```python
from build123d import *

# Parameters (mm, degrees)
F1_DEPTH = 20
F3_DEPTH = 20


with BuildPart() as f1:
    # F0 (on Top) → F1 (new body)
    with BuildSketch(Plane.XY):
        Polygon((0, 40), (0, 0), (20, 0), (20, 20), (40, 20), (40, 40), align=None)
    extrude(amount=F1_DEPTH)

    # F2 (on face) → F3 (join)
    with BuildSketch(Plane.XY.offset(20)):
        Polygon((0, 20), (20, 20), (40, 40), (0, 40), align=None)
    extrude(amount=F3_DEPTH)


solid = f1.part
```
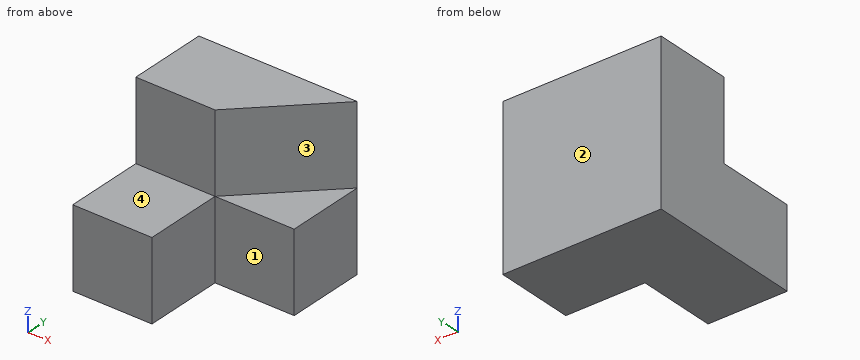
Could you check a few things on this model? Use its own coordinates, in mm. Face numbers are marked on the shaded views. A direction names the side the tool comes from. Give positions to 0.01 mm unless a question says otherwise; leave off trailing zeros. Write each loop counter-clockwise with the first axis right and the second up, starting at its lowest first coordinate (ties: lowest second). Pieces come first, ordered by that corner, then holes. Notation, with made-up numbers: (41, -7) - (67, -7) arc R25 ccw to (67, 21) - close; hole circle Ø8 at (50, 10.5). An arc over 180 degrees is marked (long way). One line per item, written item: value. Start each with the question number.
Item 1: Imagine slicing it at B-B, the plane x = 13. List the corners of the cut face in (y, z) for me, and give its area (3 significant figures).
Item 2: Imagine slicing it at D-D, the plane y = 12. List the corners of the cut face in (x, z) for me.
Item 3: Imagine slicing it at A-A, the plane y = 35. List the corners of the cut face in (x, z) for me.
Item 4: I'm going to push flat-ended pins straight in: pin 1 (6 mm diameter, centred on x = 7, z = 31, fed in from -Y); pin 2 (2 mm diameter, centred on y = 25, z = 25, fed in from +X); pin 3 (6 mm diameter, centred on y = 8, z = 12.5, fed in from +X). Where does each tip first touch, or does it pass through?
Item 5: Imagine slicing it at C-C, the plane z = 34. List the corners of the cut face in (x, y) for me, and give its area (3 significant figures).
Item 6: Which directions (+Z, -Z, +X, -X, +Y, -Y) give clear straight access to the entire face, cutting with the end or side of a thin tool? Please do the marked faces 1, 2, 3 and 4.
Item 7: Please list where these lines run through material, in increasing order: line 1 (Z direction, x = 11, y = 3); line 2 (Y direction, x = 33, z = 5.5). Write a range as from..to.
Geometry says:
1. outline: (0, 0) - (40, 0) - (40, 40) - (20, 40) - (20, 20) - (0, 20) - close
1. area: 1,200 mm^2
2. outline: (0, 0) - (20, 0) - (20, 20) - (0, 20) - close
3. outline: (0, 0) - (40, 0) - (40, 20) - (35, 20) - (35, 40) - (0, 40) - close
4. pin 1: y = 20
4. pin 2: x = 26
4. pin 3: x = 20
5. outline: (0, 20) - (20, 20) - (40, 40) - (0, 40) - close
5. area: 600 mm^2
6. face 1: +Z, -Z, +X, -Y
6. face 2: +Z, -Z, +X, -X, +Y
6. face 3: +Z, +X, -Y
6. face 4: +Z, +X, -X, -Y
7. line 1: 0..20
7. line 2: 20..40
